Geometry: final body of the model. Coordinates: model frame, mm. A direction names the side the tool comes from. Give positions to 0.01 mm unless a question says otherwise; leave off trailing zeros. Write each loop counter-clockwise with the first axis right and the second up, starting at its lowest first coordinate (ties: lowest second). Pieces come first, ordered by that corner, then holes. Notation, with made-up numbers: (-31, 36.25) -> (21, 36.25) arc R23 cw to (21, 75.25) -> close; hole circle Ø5 at (-21, 66). An arc over 180 degrees is marked (long way). Answer as a JSON object with one key per item and string values.
Autodesk Inventor part; units mm, degrees
ref_plane "YZ Plane" through (0, 0, 0) normal (1, 0, 0) x (0, 1, 0)
ref_plane "XZ Plane" through (0, 0, 0) normal (0, 1, 0) x (-1, 0, 0)
ref_plane "XY Plane" through (0, 0, 0) normal (0, 0, 1) x (1, 0, 0)
sketch "Sketch1" plane through (0, 0, 0) normal (1, 0, 0) x (0, 1, 0)
  line L0 (0, -8.3) -> (7.6716, -8.3)
  line L1 (14, 0) -> (0, 0) construction
  line L2 (0, 0) -> (0, -8.3) construction
  line L3 (6.1716, -9.8) -> (0, -9.8)
  line L4 (0, -8.3) -> (0, -9.8)
  line L5 (25.1284, -11.1284) -> (25.1284, -14.1284)
  line L6 (25.1284, -14.1284) -> (26.6284, -14.1284)
  line L7 (14, 0) -> (22, 0)
  line L8 (25.1284, -11.1284) -> (14, 0)
  line L9 (26.6284, -14.1284) -> (26.6284, -11.1284)
  line L10 (26.6284, -11.1284) -> (22, 0)
  line L11 (7.6716, -8.3) -> (10.5, -11.1284)
  line L12 (10.5, -11.1284) -> (10.5, -14.1284)
  line L13 (10.5, -14.1284) -> (6.1716, -9.8)
  line L14 (25.1284, -11.1284) -> (10.5, -11.1284) construction
  dimension "d2" = 14
  dimension "d3" = 8.3
  dimension "d9" = 1.5
  dimension "d71" = 1.5
  dimension "d72" = 3
  dimension "d74" = 8
  dimension "d170" = 3
  dimension "d171" = 4
  dimension "d172" = 135
  dimension "d176" = 3.5
revolve "Revolution3" add sketch "Sketch1" angle 360 about axis through (0, 14, 0) along (0, -1, 0)
ref_plane "Work Plane2" through (0, 21.25, 0) normal (0, -1, 0) x (1, 0, 0)
sketch "Sketch13" plane through (0, 21.25, 0) normal (0, -1, 0) x (1, 0, 0)
  arc A0 (-13.9739, 0.8547) -> (-13.9739, -0.8547) centre (0, 0) ccw
  line L0 (0, 0) -> (-13.9739, -0.8547) construction
  line L1 (0, 0) -> (14, 0) construction
  line L2 (0, 0) -> (-13.9739, 0.8547) construction
  arc A1 (-10.4804, 0.641) -> (-10.4804, -0.641) centre (0, 0) ccw
  line L3 (0, 0) -> (-10.4804, 0.641) construction
  line L4 (0, 0) -> (-10.4804, -0.641) construction
  line L5 (-13.9739, -0.8547) -> (-10.4804, -0.641)
  line L6 (-13.9739, 0.8547) -> (-10.4804, 0.641)
  line L7 (0, 2.675) -> (0, -2.675)
  arc A2 (13.9739, -0.8547) -> (13.9739, 0.8547) centre (0, 0) ccw
  arc A3 (10.4804, -0.641) -> (10.4804, 0.641) centre (0, 0) ccw
  line L8 (13.9739, -0.8547) -> (10.4804, -0.641)
  line L9 (13.9739, 0.8547) -> (10.4804, 0.641)
  line L10 (-1.7678, 1.7678) -> (1.7678, -1.7678)
  line L11 (-1.7678, 1.7678) -> (3.2322, 1.7678) construction
  arc A4 (0.8547, 13.9739) -> (-0.8547, 13.9739) centre (0, 0) ccw
  arc A5 (0.641, 10.4804) -> (-0.641, 10.4804) centre (0, 0) ccw
  line L12 (0.8547, 13.9739) -> (0.641, 10.4804)
  line L13 (-0.8547, 13.9739) -> (-0.641, 10.4804)
  arc A6 (-0.8547, -13.9739) -> (0.8547, -13.9739) centre (0, 0) ccw
  arc A7 (-0.641, -10.4804) -> (0.641, -10.4804) centre (0, 0) ccw
  line L14 (-0.8547, -13.9739) -> (-0.641, -10.4804)
  line L15 (0.8547, -13.9739) -> (0.641, -10.4804)
  point P0 (0, 0)
  dimension "d150" = 14
  dimension "d151" = 176.5
  dimension "d152" = 7
  dimension "d153" = 10.5
  dimension "d154" = 7
  dimension "d155" = 5.35
  dimension "d156" = 5
  dimension "d157" = 45
extrude "Extrusion7" add sketch "Sketch13" along normal blind 14.25 and the other way blind 4.75
properties part number "soundconev4"
Q1. Mould query, pull axis Y, two halves, no side actions, for faces 1 (the conical face through (-0.952, 17.169, -3.023)), 2 (the flat face through (0, 7, 12)), 3 (the flat face through (13.1, 8, -0.8)). Classes: pulls with the +Y half, pulls with the -Y half, needs draft (parallel to the pull), parting line crosses it, or undercut.
Values:
{"face 1": "undercut", "face 2": "pulls with the -Y half", "face 3": "needs draft"}
Q2. Cut plane C-C (x = 6). State how many separate pieces and enclosed holes the cut face has, and give its area (3 significant figures).
Values:
{"separate pieces": "3", "enclosed holes": "0", "area": "127 mm²"}
Q3. First-contact query: P1, Ø1.4, axis at x = -11.5, z = 0, coming from the -Y side; P2, Ø1, axis at y = 9, z = -9.5, coming from the +X side; P3, Ø13.5, axis at x = 0, z = 0, coming from the +Y side. Flat tips, straight axial feed; report the tip coordinate or a pass-through.
Values:
{"P1": "y = 7", "P2": "x = 9.23", "P3": "y = 24.81"}
Q4. Cut plane A-A (y = 15.5). Return the cut outline in (x, z), and give its area (3 significant figures).
Values:
{"outline": "(-13.97, -0.85) -> (-10.48, -0.64) arc R10.5 cw to (-10.48, 0.64) -> (-13.97, 0.85) arc R14 ccw to start; circle Ø3 at (0, 0); (-0.85, -13.97) arc R14 ccw to (0.85, -13.97) -> (0.64, -10.48) arc R10.5 cw to (-0.64, -10.48) -> close; (-0.85, 13.97) -> (-0.64, 10.48) arc R10.5 cw to (0.64, 10.48) -> (0.85, 13.97) arc R14 ccw to start; (10.48, -0.64) -> (13.97, -0.85) arc R14 ccw to (13.97, 0.85) -> (10.48, 0.64) arc R10.5 cw to start", "area": "28.0 mm²"}
Q5. Set-up query: faces 4 (the flat face through (13.1, 8, 0.8)), 5 (the flat face through (-0.8, 8, -13.1)), 6 (the flat face through (0.8, 8, -13.1)), 7 (the cylindrical face through (8.103, 3.89, 1.799)), 8 (the cylindrical face through (-10.5, 17.3, 0)). Return all of +Z, -Z, +X, -X, +Y, -Y with unobstructed straight access to the full face (end or side cutting, diameter ignored); none if empty.
Values:
{"face 4": "+Z, -Y", "face 5": "-X, -Y", "face 6": "+X, -Y", "face 7": "-Y", "face 8": "none"}
Q6. Material intervals for L1, parallel to X at y = 2.75, z = 0; L2, parallel to Y at x = -12.25, z = 5.5; L3, parallel to Y at x = -6.75, z = -9.5, sorted ascending. Write a range as from..to.
Values:
{"L1": "-9.8..-8.3, 8.3..9.8", "L2": "9.8..10.5, 25.13..26.63", "L3": "8.03..10.5, 25.13..26.63"}
Q7. Cut plane B-B (y = 12.25). Return the cut outline in (x, z).
Values:
{"outline": "(-13.97, -0.85) -> (-10.48, -0.64) arc R10.5 cw to (-10.48, 0.64) -> (-13.97, 0.85) arc R14 ccw to start; (-0.85, -13.97) arc R14 ccw to (0.85, -13.97) -> (0.64, -10.48) arc R10.5 cw to (-0.64, -10.48) -> close; (-0.85, 13.97) -> (-0.64, 10.48) arc R10.5 cw to (0.64, 10.48) -> (0.85, 13.97) arc R14 ccw to start; (10.48, -0.64) -> (13.97, -0.85) arc R14 ccw to (13.97, 0.85) -> (10.48, 0.64) arc R10.5 cw to start"}
